from build123d import *

# Parameters (mm, degrees)
SKETCH1_R                     = 3.6195
SKETCH1_R_2                   = 4.7625
SKETCH1_R_3                   = 1.6999966
BOSS_EXTRUDE1_DEPTH           = 6.35
SKETCH12_W                    = 6.35
SKETCH12_H                    = 6.1722
BOSS_EXTRUDE3_DEPTH           = 1.0668
CUT_EXTRUDE1_DEPTH            = 146.254081268
TAP_DRILL_FOR_6_32_TAP4_D     = 2.7051
TAP_DRILL_FOR_6_32_TAP3_D     = 2.7051
TAP_DRILL_FOR_6_32_TAP3_DEPTH = 10.16
TAP_DRILL_FOR_6_32_TAP3_TIP   = 0.81269403
SKETCH20_W                    = 6.35
SKETCH20_H                    = 13.543293675
SKETCH20_H_2                  = 12.7
CUT_EXTRUDE2_DEPTH            = 3.175
SKETCH21_W                    = 6.35
SKETCH21_H                    = 9.525
BOSS_EXTRUDE4_DEPTH           = 3.175


with BuildPart() as part:
    # Sketch1 → Boss-Extrude1 (new body)
    with BuildSketch(Plane(origin=(0, 0, 0), x_dir=(0, 0, -1), z_dir=(1, 0, 0))):
        Polygon((0, 0), (-14.664696837, 25.4), (-128.210303163, 25.4), (-142.875, 0), align=None)
        with Locations((-110.998, 12.7)):
            Circle(SKETCH1_R, mode=Mode.SUBTRACT)
        with Locations((-31.877, 12.7)):
            Circle(SKETCH1_R_2, mode=Mode.SUBTRACT)
        with Locations((-102.4979916, 12.7)):
            Circle(SKETCH1_R_3, mode=Mode.SUBTRACT)
        with Locations((-119.4980084, 12.7)):
            Circle(SKETCH1_R_3, mode=Mode.SUBTRACT)
    extrude(amount=BOSS_EXTRUDE1_DEPTH)

    # Sketch12 → Boss-Extrude3 (add)
    with BuildSketch(Plane(origin=(0, 0, 0), x_dir=(-1, 0, 0), z_dir=(0, 0.49999999999999806, -0.8660254037844398))):
        with Locations((-3.175, 7.9375)):
            Rectangle(SKETCH12_W, SKETCH12_H)
    boss_extrude3 = extrude(amount=BOSS_EXTRUDE3_DEPTH)

    # Sketch19 → Cut-Extrude1 (cut, through all)
    with BuildSketch(Plane.ZY):
        Polygon((92.930922513, 20.6375), (39.8145, 20.6375), (39.8145, 6.079337508), align=None)
        Polygon((97.7354916, 4.7625), (97.7354916, 19.320662492), (44.619069087, 4.7625), align=None)
        Polygon((23.9395, 20.6375), (23.9395, 4.7625), (10.081979076, 4.7625), (19.247414599, 20.6375), align=None)
    extrude(amount=-CUT_EXTRUDE1_DEPTH, mode=Mode.SUBTRACT)

    # Tap Drill for #6-32 Tap4 (through all)
    with Locations(Plane(origin=(0, 25.4, 0), x_dir=(1, 0, 0), z_dir=(0, 1, 0))):
        with Locations((3.175, -110.998), (3.175, -31.877)):
            Hole(TAP_DRILL_FOR_6_32_TAP4_D / 2)

    # Tap Drill for #6-32 Tap3
    with Locations(Plane(origin=(0, 0, 0), x_dir=(-1, 0, 0), z_dir=(0, -1, 0))):
        with Locations((-3.175, -130.175), (-3.175, -12.7)):
            Hole(TAP_DRILL_FOR_6_32_TAP3_D / 2, depth=TAP_DRILL_FOR_6_32_TAP3_DEPTH)
            with Locations((0, 0, -(TAP_DRILL_FOR_6_32_TAP3_DEPTH + TAP_DRILL_FOR_6_32_TAP3_TIP / 2))):  # 118° drill point
                Cone(0, TAP_DRILL_FOR_6_32_TAP3_D / 2, TAP_DRILL_FOR_6_32_TAP3_TIP, mode=Mode.SUBTRACT)

    # Sketch15 → Tap Drill for #6-32 Tap2 (revolve, cut)
    with BuildSketch(Plane(origin=(3.175, 17.795609612, 10.2743), x_dir=(0, 0.8660254037844398, 0.49999999999999806), z_dir=(1, 0, 0))):
        Polygon((0, 0), (0, 8.43269403), (1.35255, 7.62), (1.35255, 0), align=None)
    tap_drill_for_6_32_tap2 = revolve(axis=Axis((3.175, 20.970609612, 4.775038686), (0, -0.499999999999998, 0.8660254037844398)), mode=Mode.SUBTRACT)

    # Sketch20 → Cut-Extrude2 (cut)
    with BuildSketch(Plane(origin=(0, 0, 0), x_dir=(-1, 0, 0), z_dir=(0, 0.49999999999999806, -0.8660254037844398))):
        with Locations((-3.175, 17.795246838)):
            Rectangle(SKETCH20_W, SKETCH20_H)
        with Locations((-3.175, -1.4986)):
            Rectangle(SKETCH20_W, SKETCH20_H_2)
    cut_extrude2 = extrude(amount=-CUT_EXTRUDE2_DEPTH, mode=Mode.SUBTRACT)

    # Mirror1: Boss-Extrude3, Tap Drill for #6-32 Tap2, Cut-Extrude2 across plane
    add(boss_extrude3.mirror(Plane(origin=(0, 0, 71.4375), x_dir=(1, 0, 0), z_dir=(0, 0, -1))))
    add(tap_drill_for_6_32_tap2.mirror(Plane(origin=(0, 0, 71.4375), x_dir=(1, 0, 0), z_dir=(0, 0, -1))), mode=Mode.SUBTRACT)
    add(cut_extrude2.mirror(Plane(origin=(0, 0, 71.4375), x_dir=(1, 0, 0), z_dir=(0, 0, -1))), mode=Mode.SUBTRACT)

    # Sketch21 → Boss-Extrude4 (add)
    with BuildSketch(Plane(origin=(0, 25.4, 0), x_dir=(1, 0, 0), z_dir=(0, 1, 0))):
        with Locations((3.175, -48.129196837)):
            Rectangle(SKETCH21_W, SKETCH21_H)
        with Locations((3.175, -94.872803163)):
            Rectangle(SKETCH21_W, SKETCH21_H)
    extrude(amount=BOSS_EXTRUDE4_DEPTH)


solid = part.part
Here's how the part is built. I have some questions about the finished solid (model axes, mm). A direction names the side the tool comes from. Coordinates: 2 decimals unless noted, no trailing zeros. Order: outer loops, then holes, each group sorted by start corner. A loop starts at its lowest first (then second) coordinate and runs counter-clockwise, first axis right, second up. Notation, with made-up numbers: M 10.5,87 L 58.5,87 A33 ccw 58.5,116 Z; hole C -2,23.5 d1. An arc over 180 degrees is marked long. Answer as CSV lines item,"result".
Item 1: On a 3-axis mill with a long thin cutter (end or side, diameter ignored), from which of +Z, -Z, +X, -X, +Y, -Y can I reach the whole of each face in a straight line? I mean faces 4 (the face through (2.88, 2.41, 14.02)), 5 (the face through (3, 20.638, 22)), 6 (the face through (3.22, 3.66, 3.36)). Say none if no direction works.
Results found:
face 4,"-Y"
face 5,"+X, -X"
face 6,"-Z, +X, -X"
Item 2: Imagine slicing it at B-B on z = 72. Write out the boundary of the cut face in (x, y).
Results found:
outline,"M 0,0 L 6.35,0 L 6.35,4.76 L 0,4.76 Z; M 0,12.27 L 6.35,12.27 L 6.35,14.9 L 0,14.9 Z; M 0,20.64 L 6.35,20.64 L 6.35,25.4 L 0,25.4 Z"
Item 3: We'd pull the mould along Y, two halves only. Please class faces 1 (the face through (3, 0, 72)), 2 (the face through (3.22, 1.33, 138.44)), 3 (the face through (3, 27, 99.635)): +Y half, -Y half, draft (parallel to the pull), parting line (faces both ways), or undercut.
Results found:
face 1,"-Y half"
face 2,"undercut"
face 3,"draft"
Item 4: Imagine slicing it at C-C on z = 50. Give the number of separate pieces and of enclosed holes in the cut face, plus the area to 3 significant figures.
Results found:
separate pieces,"3"
enclosed holes,"0"
area,"97.4 mm2"
Item 5: For pin 1 (2.5 mm diameter, centred on x = 2.5, y = 27, fed in from +Z); pin 2 (1.6 mm diameter, centred on x = 3.175, z = 12.7, fed in from +Y); pin 3 (1.5 mm diameter, centred on x = 0.5, y = 13, fed in from +Z); pin 4 (2 mm diameter, centred on x = 3.175, z = 31.877, fed in from -Y), each with a flat end and sliding along its axis, tell me the tip position at first contact or that it passes through.
Results found:
pin 1,"z = 99.64"
pin 2,"y = 23.38"
pin 3,"z = 132.14"
pin 4,"through"
Item 6: If I drill on line 1 (Z direction, x = 3.5, y = 2); line 2 (Y direction, x = 2, z = 18.5); line 3 (Y direction, x = 3.75, z = 60), over which ranges is the centre line in solid material (lowest first)?
Results found:
line 1,"4.82 to 11.39, 14.01 to 30.56, 33.19 to 109.69, 112.31 to 128.86, 131.49 to 138.05"
line 2,"0 to 4.76, 19.34 to 25.4"
line 3,"0 to 4.76, 8.98 to 11.61, 20.64 to 25.4"
